CAD build for the part. Positions are in the model's coordinates, mm. Give positions to 0.01 mm unless a question says otherwise; leave off trailing zeros. Loops run counter-clockwise (first coordinate to the right, second up) from the corner with the lowest first, then second, coordinate; pieces in that order, holes last. Notation, with made-up numbers: M -5,12 L 33,12 A5 cw 33,16 Z; hole C -34,-1.75 d5. An arc over 180 degrees is marked long. Answer as CSV lines item,"result".
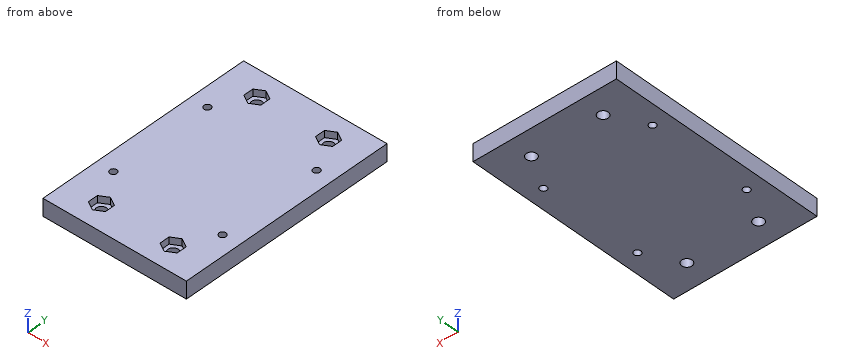
```python
from build123d import *

# Parameters (mm, degrees)
SKETCH_1_W          = 42
SKETCH_1_H          = 64
EXTRUDE_1_DEPTH     = 5
CUT_EXTRUDE_1_DEPTH = 2
SKETCH_4_R          = 1.5
CUT_EXTRUDE_2_DEPTH = 77.609398901
SKETCH_5_R          = 1
CUT_EXTRUDE_3_DEPTH = 5


with BuildPart() as part:
    # 스케치1 → 보스-돌출1 (new body)
    with BuildSketch(Plane.XY):
        with Locations((21, -32)):
            Rectangle(SKETCH_1_W, SKETCH_1_H)
    extrude(amount=EXTRUDE_1_DEPTH)

    # 스케치2 → 컷-돌출1 (cut)
    with BuildSketch(Plane.XY.offset(5)):
        Polygon((10.5, -4.313248654), (10.5, -10.086751346), (8, -8.643375673), (8, -5.756624327), align=None)
        Polygon((13, -5.756624327), (10.5, -4.313248654), (10.5, -10.086751346), (13, -8.643375673), align=None)
        Polygon((31.5, -4.313248654), (31.5, -10.086751346), (29, -8.643375673), (29, -5.756624327), align=None)
        Polygon((34, -5.756624327), (31.5, -4.313248654), (31.5, -10.086751346), (34, -8.643375673), align=None)
        Polygon((10.5, -53.913248654), (10.5, -59.686751346), (8, -58.243375673), (8, -55.356624327), align=None)
        Polygon((13, -55.356624327), (10.5, -53.913248654), (10.5, -59.686751346), (13, -58.243375673), align=None)
        Polygon((31.5, -53.913248654), (31.5, -59.686751346), (29, -58.243375673), (29, -55.356624327), align=None)
        Polygon((34, -55.356624327), (31.5, -53.913248654), (31.5, -59.686751346), (34, -58.243375673), align=None)
    extrude(amount=-CUT_EXTRUDE_1_DEPTH, mode=Mode.SUBTRACT)

    # 스케치4 → 컷-돌출2 (cut, through all)
    with BuildSketch(Plane.XY.offset(3)):
        with Locations((10.5, -7.2)):
            Circle(SKETCH_4_R)
        with Locations((31.5, -7.2)):
            Circle(SKETCH_4_R)
        with Locations((31.5, -56.8)):
            Circle(SKETCH_4_R)
        with Locations((10.5, -56.8)):
            Circle(SKETCH_4_R)
    extrude(amount=-CUT_EXTRUDE_2_DEPTH, mode=Mode.SUBTRACT)

    # 스케치5 → 컷-돌출3 (cut)
    with BuildSketch(Plane.XY.offset(5)):
        with Locations((5, -17)):
            Circle(SKETCH_5_R)
        with Locations((37, -17)):
            Circle(SKETCH_5_R)
        with Locations((5, -47)):
            Circle(SKETCH_5_R)
        with Locations((37, -47)):
            Circle(SKETCH_5_R)
    extrude(amount=-CUT_EXTRUDE_3_DEPTH, mode=Mode.SUBTRACT)


solid = part.part
```
Q1. Cut at C-C (y = -56.8). Write the cut outline in (x, z).
Solution:
outline,"M 0,0 L 9,0 L 9,3 L 8,3 L 8,5 L 0,5 Z; M 12,0 L 30,0 L 30,3 L 29,3 L 29,5 L 13,5 L 13,3 L 12,3 Z; M 33,0 L 42,0 L 42,5 L 34,5 L 34,3 L 33,3 Z"
Q2. Pin check, flat tips, straight feed: P1, Ø2, axis at y = -6.5, z = 4, coming from the -X side; P2, Ø3.5, axis at x = 31.5, y = -7.2, coming from the +Z side. Stop position of each tip, or through.
Solution:
P1,"stops at x = 0"
P2,"stops at z = 3"
Q3. Cut at D-D (y = -47). Write the cut outline in (x, z).
Solution:
outline,"M 0,0 L 4,0 L 4,5 L 0,5 Z; M 6,0 L 36,0 L 36,5 L 6,5 Z; M 38,0 L 42,0 L 42,5 L 38,5 Z"
Q4. Wall check: line 1 (Y direction, x = 37, z = 3.6); line 2 (X direction, y = -56.5, z = 3.8); line 3 (Y direction, x = 11, z = 2.85). Give the ranges that are in metal, low to high. Write a range as [from, to].
Solution:
line 1,"y = [-64, -48], [-46, -18], [-16, 0]"
line 2,"x = [0, 8], [13, 29], [34, 42]"
line 3,"y = [-64, -58.21], [-55.39, -8.61], [-5.79, 0]"
Q5. Cut at A-A (z = 0.75). Give the number of separate pieces and of enclosed holes in the cut face, and give its area (3 significant figures).
Solution:
separate pieces,"1"
enclosed holes,"8"
area,"2,650 mm²"
Q6. Cut at B-B (x = 37). Write the cut outline in (y, z), and give its area (3 significant figures).
Solution:
outline,"M -64,0 L -48,0 L -48,5 L -64,5 Z; M -46,0 L -18,0 L -18,5 L -46,5 Z; M -16,0 L 0,0 L 0,5 L -16,5 Z"
area,"300 mm²"
